Geometry: final body of the model. Coordinates: model frame, mm. A direction names the side the tool comes from. Give positions to 0.01 mm unless a question says otherwise; leave off trailing zeros. Order: outer loops, then holes, each group sorted by start corner. A loop starts at its lowest first (then second) coordinate and runs counter-clockwise, first axis right, second up. Notation, with made-up numbers: (84, 63) -> (117, 63) arc R14 ccw to (117, 79) -> close; hole circle Ø6 at (36.5, -2). An arc over 180 degrees is marked (long way). One line per question, with ' | ' between items. Start each with the question number.
(1) Set-up query: faces 4 (the face through (13, 13, -19.05)), 5 (the face through (-10.18, 14.63, -9.39)). Return all of +Z, -Z, +X, -X, +Y, -Y with unobstructed straight access to the full face (end or side cutting, diameter ignored); none if empty.
(2) Section A-A (z = -10.75). Return loops of the section in (x, y) (3 decimals).
(3) Mould query, pull axis X, two halves, no side actions, for faces 1 (the face through (11.2, 15.5, -9.4)), 2 (the face through (-13, 13, -19.05)), 3 (the face through (-1.117, 50.788, 1.565)). Classes: +X half, -X half, draft (parallel to the pull), parting line (faces both ways), or undercut.
(4) Section B-B (x = -12.7). Return loops of the section in (y, z) (3 decimals).
(5) Section C-C (y = 12.7). Return loops of the section in (x, z) (3 decimals), then the cut area to 3 significant figures.
(6) Section D-D (x = 0). Return loops of the section in (y, z) (3 decimals), then the cut area to 3 significant figures.
(7) First-contact query: pin 1 Ø8 at (y, z) = (24, 0) entering from -X; pin 2 Ø2 at (x, y) = (11.5, 27.5) entering from -Z; pin 3 Ø2 at (y, z) = (27, -2) entering from +X. Flat tips, straight axial feed; report the tip coordinate or a pass-through.
(8) Ray query, L1, parallel to Z at x = 13, y = 46.5 (3 decimals); L2, parallel to X at y = 14, z = -3; L3, parallel to Y at x = -15, z = -1.75. Return the intervals inside material, ascending.
Autodesk Inventor part; units mm, degrees
ref_plane "YZ Plane" through (0, 0, 0) normal (1, 0, 0) x (0, 1, 0)
ref_plane "XZ Plane" through (0, 0, 0) normal (0, 1, 0) x (-1, 0, 0)
ref_plane "XY Plane" through (0, 0, 0) normal (0, 0, 1) x (1, 0, 0)
sketch "Sketch1" plane through (0, 0, 0) normal (0, 0, 1) x (1, 0, 0)
  arc A0 (50.8, 0) -> (-50.8, 0) centre (0, 0) ccw
  line L0 (0, 0) -> (50.8, 0)
  line L1 (0, 0) -> (-50.8, 0)
  dimension "d0" = 101.6
extrude "Extrusion1" add sketch "Sketch1" along normal blind 3.175
sketch "Sketch4" plane through (0, 0, 0) normal (0, 0, -1) x (-1, 0, 0)
  line L0 (0, 0) -> (0, 12.7) construction
  line L1 (0, 12.7) -> (12.7, 12.7) construction
  circle A0 centre (12.7, 12.7) radius 3.175
  circle A1 centre (-12.7, 12.7) radius 3.175
  dimension "d15" = 12.7
  dimension "d16" = 12.7
  dimension "d17" = 6.35
extrude "Extrusion5" add sketch "Sketch4" along normal blind 19.05
sketch "Sketch5" plane through (0, 0, 3.175) normal (0, 0, 1) x (1, 0, 0)
  line L0 (-2.5936, 17.577) -> (2.4467, 17.6618)
  line L1 (2.4467, 17.6618) -> (5.0403, 13.3391)
  line L2 (5.0403, 13.3391) -> (2.5936, 8.9317)
  line L3 (2.5936, 8.9317) -> (-2.4467, 8.8469)
  line L4 (-2.4467, 8.8469) -> (-5.0403, 13.1696)
  line L5 (-5.0403, 13.1696) -> (-2.5936, 17.577)
  line L6 (0, 0) -> (0, 21.7215) construction
  point P0 (0, 13.2543)
  dimension "d22" = 4.3656
  dimension "d23" = 0
properties part number "Rear"
Response:
1) face 4: -Z, +X, -X, +Y, -Y | face 5: -Z
2) outline: circle Ø6.35 at (-12.7, 12.7); circle Ø6.35 at (12.7, 12.7)
3) face 1: undercut | face 2: draft | face 3: parting line
4) outline: (0, 0) -> (9.525, 0) -> (9.525, -19.05) -> (15.875, -19.05) -> (15.875, 0) -> (49.187, 0) -> (49.187, 3.175) -> (0, 3.175) -> close
5) outline: (-49.187, 0) -> (-15.875, 0) -> (-15.875, -19.05) -> (-9.525, -19.05) -> (-9.525, 0) -> (9.525, 0) -> (9.525, -19.05) -> (15.875, -19.05) -> (15.875, 0) -> (49.187, 0) -> (49.187, 3.175) -> (-49.187, 3.175) -> close | area: 554 mm^2
6) outline: (0, 0) -> (50.8, 0) -> (50.8, 3.175) -> (0, 3.175) -> close | area: 161 mm^2
7) pin 1: stops at x = -46.7 | pin 2: stops at z = 0 | pin 3: passes through
8) L1: z = 0 to 3.175 | L2: x = -15.6 to -9.8, 9.8 to 15.6 | L3: y = 10.51 to 14.89
